Job drawing, mm, ordinate dimensions from the low corner. One solid piece. Coordinates: 2 decimals unless noted, no trailing zeros. Write each loop counter-clockwise with the first axis right and the second up, starting at its lowest first coordinate (ties: lowest second). Pieces come first, ordered by that corner, then holes. Notation, with made-up numbers: (-24, -24.5) -> (-8, -24.5) arc R28 cw to (-8, 4.5) -> close; hole circle Ø11 at (33.25, 49.25). An arc over 180 degrees is marked (long way). One line per question, with ' | ' between items. Start each with the question number.
Item 1: Probe probe 1 along Y at (x, z) = (4, 35.5); probe 2 along X at (y, z) = (9, 10); probe 3 along Y at (x, z) = (35.5, 51). List the from-to ranges inside material, lowest first. Write a range as [from, to].
Item 2: Saw through at A-A (z = 61). List the corners of the cut face in (x, y), and give its area (3 significant figures).
Item 3: Pin check, flat tips, straight feed: pin 1 (6 mm diameter, centred on y = 12.5, z = 9, fed in from +X); pin 2 (2 mm diameter, centred on x = 10, z = 20.5, fed in from -Y); pin 3 (2 mm diameter, centred on y = 21.5, z = 65, fed in from -X). Stop position of each tip, or through.
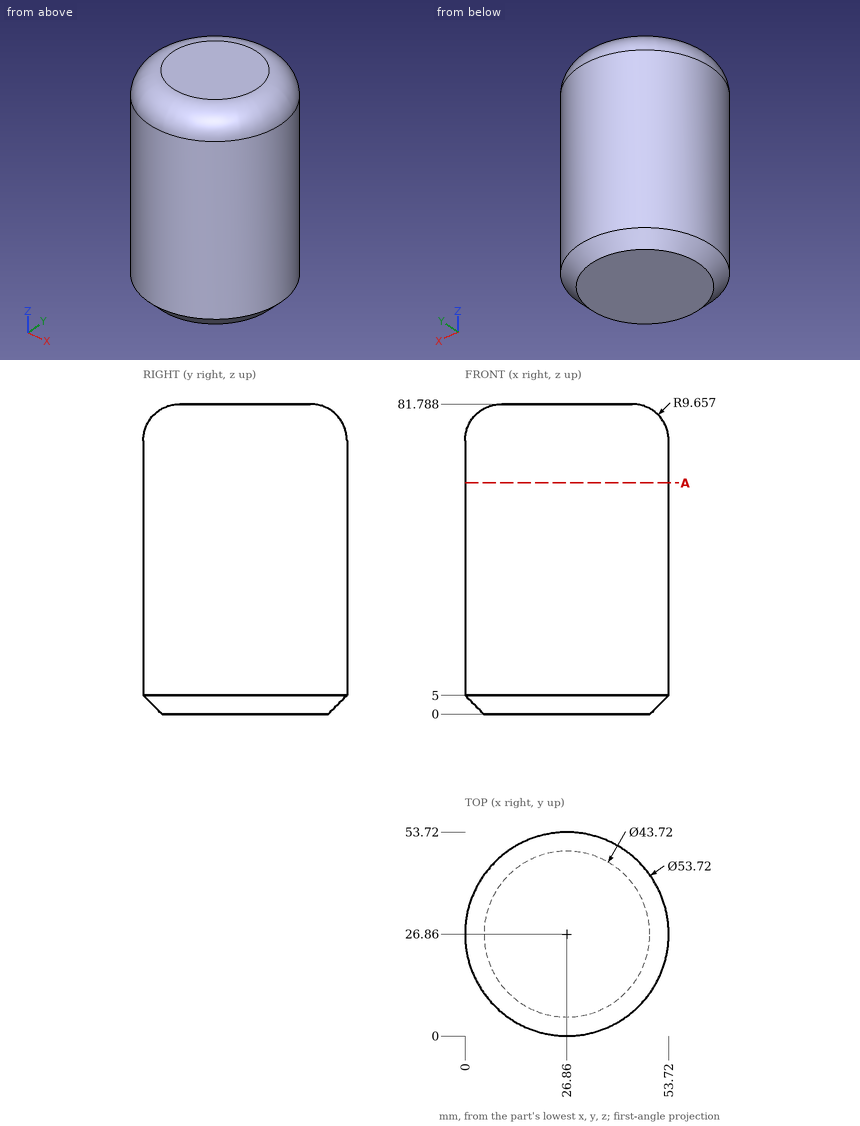
From the geometry:
1) probe 1: [12.76, 40.96] | probe 2: [6.8, 46.92] | probe 3: [1.43, 52.29]
2) outline: circle Ø53.72 at (26.86, 26.86) | area: 2,270 mm2
3) pin 1: x = 51.2 | pin 2: y = 5.18 | pin 3: x = 0.36
